Print and shaded views of the part. All mm, measured from the part's lowest x, y and z. A direction names the side the tool comes from. Round coordinates to 2 decimals unless told otherwise and drop trailing zeros. Order: outer loops, then holes, each group sorted by start corner. A loop starts at its lowest first (then second) coordinate and runs counter-clockwise, first axis right, second up. Notation, with made-up numbers: (33.5, -40) - (88.5, -40) arc R20 cw to (88.5, -1) - close; hole circle Ø8 at (45.5, 76). An arc over 180 degrees is marked (long way). Return JSON: item names as keys, results as strings. Group by question number.
Item 1: Tool access for the marked faces 1 and 2: list every direction of +Z, -Z, +X, -X, +Y, -Y with a clear straight run to the whole face (end or side of a thin tool).
Item 2: Probe probe 1 along X at (y, z) = (28.5, 19); probe 2 along Z at (x, y) = (38.5, 8); probe 3 along Y at (x, z) = (34, 13). List the from-to ranges inside material, lowest first.
Item 3: Saw through at B-B on y = 33. List the corners of the cut face in (x, z).
Item 4: Saw through at A-A on z = 9. List the corners of the cut face in (x, y), and give its area (3 significant figures).
Item 5: Saw through at C-C on x = 35.5. List the corners of the cut face in (y, z), and give its area (3 significant figures).
Item 6: Drop flat-ended pins along their axis: pin 1 (10 mm diameter, centred on x = 18, z = 32.5, fed in from +Y); pin 2 (1 mm diameter, centred on x = 19, z = 7.5, fed in from -Y); pin 3 (2 mm diameter, centred on x = 13, y = 18, fed in from -Z). Give the stop position or say it passes through.
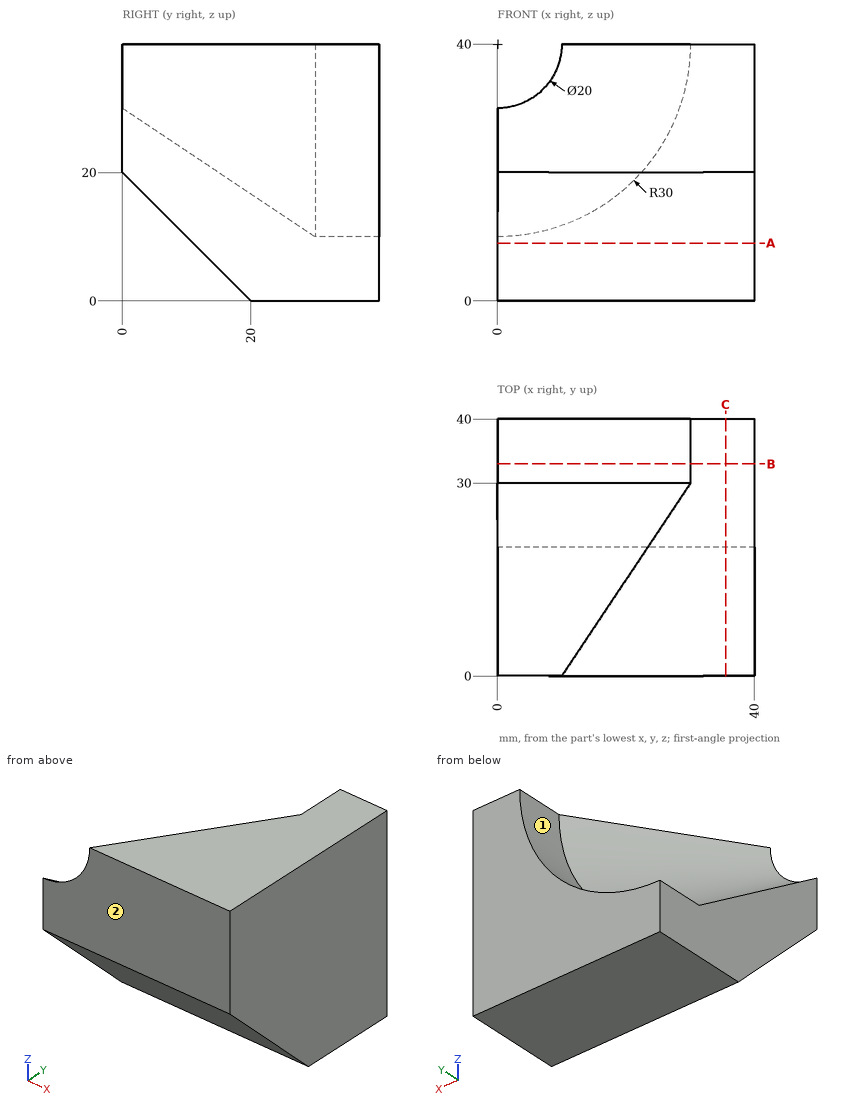
Filled in:
{
 "1": {"face 1": "+Z, -X, +Y", "face 2": "+Z, -Z, +X, -X, -Y"},
 "2": {"probe 1": "x = 20 to 40", "probe 2": "z = 12 to 40", "probe 3": "y = 7 to 40"},
 "3": {"outline": "(0, 0) - (40, 0) - (40, 40) - (30, 40) arc R30 cw to (0, 10) - close"},
 "4": {"outline": "(0, 11) - (40, 11) - (40, 40) - (0, 40) - close", "area": "1,160 mm^2"},
 "5": {"outline": "(0, 20) - (20, 0) - (40, 0) - (40, 40) - (0, 40) - close", "area": "1,400 mm^2"},
 "6": {"pin 1": "stops at y = 21.75", "pin 2": "stops at y = 12", "pin 3": "stops at z = 1"}
}
